CAD build for the part. Positions are in the model's coordinates, mm. Face numbers are marked on the shaded views. A direction names the side the tool comes from. Give positions to 0.01 mm unless a question says otherwise; leave off trailing zeros. Order: outer loops, then holes, each group sorted by start corner. A loop starts at its lowest first (then second) coordinate and runs counter-clockwise, first axis right, second up.
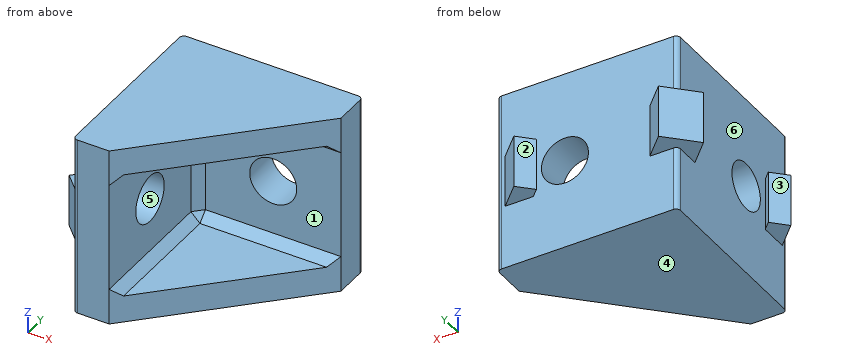
```python
from build123d import *

# Parameters (mm, degrees)
EXTRUDE_1_DEPTH     = 10
EXTRUDE_2_DEPTH     = 3
SKETCH_3_R          = 2.6
CUT_EXTRUDE_1_DEPTH = 25.738633754
SKETCH_4_R          = 2.6
CUT_EXTRUDE_2_DEPTH = 25.738633754
EXTRUDE_START       = -10
EXTRUDE_3_DEPTH     = 2.9
FILLET_1_R          = 0.5
CHAMFER_1_SIZE      = 1


with BuildPart() as part:
    # Эскиз1 → Бобышка-Вытянуть1 (new, symmetric)
    with BuildSketch(Plane.XY):
        Polygon((0, 0), (0, -16), (-4, -16), (-4, 4), (16, 4), (16, 0), align=None)
    extrude(amount=EXTRUDE_1_DEPTH, both=True)

    # Эскиз2 → Бобышка-Вытянуть2 (add)
    with BuildSketch(Plane.XY.offset(10)):
        Polygon((0, -16), (0, 0), (16, 0), align=None)
    extrude_2 = extrude(amount=-EXTRUDE_2_DEPTH)

    # Зеркальное отражение1: Бобышка-Вытянуть2 across plane
    add(extrude_2.mirror(Plane.XY))

    # Эскиз3 → Вырез-Вытянуть1 (cut, through all)
    with BuildSketch(Plane(origin=(0, 0, 0), x_dir=(0, 0, -1), z_dir=(1, 0, 0))):
        with Locations((0, -8.5)):
            Circle(SKETCH_3_R)
        with Locations((20, -8.5)):
            Circle(SKETCH_3_R)
        with Locations((20, 11.5)):
            Circle(SKETCH_3_R)
        with Locations((0, 11.5)):
            Circle(SKETCH_3_R)
    extrude(amount=-CUT_EXTRUDE_1_DEPTH, mode=Mode.SUBTRACT)

    # Эскиз4 → Вырез-Вытянуть2 (cut, through all)
    with BuildSketch(Plane.XZ):
        with Locations((8.5, 0)):
            Circle(SKETCH_4_R)
        with Locations((-11.5, 0)):
            Circle(SKETCH_4_R)
        with Locations((-11.5, 20)):
            Circle(SKETCH_4_R)
        with Locations((8.5, 20)):
            Circle(SKETCH_4_R)
    extrude(amount=-CUT_EXTRUDE_2_DEPTH, mode=Mode.SUBTRACT)

    # Эскиз5 → Бобышка-Вытянуть3 (add, symmetric)
    with BuildSketch(Plane.XY.offset(10).offset(EXTRUDE_START)):
        Polygon((-0.888730163, 4), (-3.292893219, 6.404163056), (-6.404163056, 3.292893219), (-4, 0.888730163), (-4, 4), align=None)
        Polygon((16, 3.111269837), (12.707106781, 6.404163056), (11.151471863, 4.848528137), (16, 0), align=None)
        Polygon((-4.848528137, -11.151471863), (0, -16), (-3.111269837, -16), (-6.404163056, -12.707106781), align=None)
    extrude(amount=EXTRUDE_3_DEPTH, both=True)

    # Скругление1
    fillet_1_edges = [part.edges().sort_by_distance(p)[0] for p in [
        (-4, -16, 0),
        (-4, 4, 6.45),
        (16, 4, 0),
        (-4, 4, -6.45),
    ]]
    fillet(fillet_1_edges, radius=FILLET_1_R)

    # Фаска1
    chamfer_1_edges = [part.edges().sort_by_distance(p)[0] for p in [
        (0, 0, 0),
        (0, -8, 7),
        (8, 0, 7),
        (8, 0, -7),
        (0, -8, -7),
    ]]
    chamfer(chamfer_1_edges, length=CHAMFER_1_SIZE)


solid = part.part
```
Item 1: Tool access for the marked faces 1, 2 and 3: list every direction of +Z, -Z, +X, -X, +Y, -Y with a clear straight run to the whole face (end or side of a thin tool).
Item 2: Slice it at B-B (z = 1). Give the cut face in (x, y).
Item 3: Drop flat-ended pins along their axis: pin 1 Ø4 at (x, z) = (6, -8) entering from +Y; pin 2 Ø0.7 at (x, y) = (13, 5.5) entering from -Z; pin 3 Ø8 at (y, z) = (-6, 6) entering from +X. Give the stop position or say it passes through.
Item 4: Two-plate mould, pull along Z, no slides. Class the marked faces 4, 5 and 6: released by +Z, released by -Z, zero draft, split by the parting line, or undercut.
Item 5: Wall check: L1, parallel to Y at x = -0.85, z = 0; L2, parallel to Z at x = 8.5, y = 2.75; L3, parallel to Z at x = 10.75, y = -3.75. Give the ranges that are in metal, low to high.
Item 6: Slice it at A-A (x = 8.5). Give the cut face in (y, z), and give its area (3 significant figures).
Item 7: Slice it at D-D (y = -4). Give the cut face in (x, z), and give its area (3 significant figures).
Item 8: Slice it at C-C (y = -8.5). Give the cut face in (x, z), and give its area (3 significant figures).
A:
1. face 1: +X, -Y
1. face 2: +Z, -Z, +Y
1. face 3: +Z, -Z, -X
2. outline: (-6.4, -12.71) - (-4, -15.11) - (-4, -15.5) arc R0.5 ccw to (-3.5, -16) - (0, -16) - (0, -10.9) - (-4, -10.9) - (-4, -12) - (-4.85, -11.15) - close; (-6.4, 3.29) - (-4, 0.89) - (-4, -6.1) - (0, -6.1) - (0, -1) - (1, 0) - (6.1, 0) - (6.1, 4) - (-0.89, 4) - (-3.29, 6.4) - close; (10.9, 0) - (16, 0) - (16, 3.5) arc R0.5 ccw to (15.5, 4) - (15.11, 4) - (12.71, 6.4) - (11.15, 4.85) - (12, 4) - (10.9, 4) - close
3. pin 1: stops at y = 4
3. pin 2: stops at z = -2.9
3. pin 3: stops at x = 13.87
4. face 4: released by -Z
4. face 5: undercut
4. face 6: zero draft
5. L1: y = -16 to -11.1, -5.9 to 4
5. L2: z = -10 to -2.6, 2.6 to 10
5. L3: z = -10 to -7, 7 to 10
6. outline: (-7.5, -10) - (4, -10) - (4, -2.6) - (0, -2.6) - (0, -6) - (-1, -7) - (-7.5, -7) - close; (-7.5, 7) - (-1, 7) - (0, 6) - (0, 2.6) - (4, 2.6) - (4, 10) - (-7.5, 10) - close
6. area: 105 mm2
7. outline: (-4, -10) - (12, -10) - (12, -7) - (1, -7) - (0, -6) - (0, 6) - (1, 7) - (12, 7) - (12, 10) - (-4, 10) - close
7. area: 153 mm2
8. outline: (-4, -10) - (7.5, -10) - (7.5, -7) - (1, -7) - (0, -6) - (0, -2.6) - (-4, -2.6) - close; (-4, 2.6) - (0, 2.6) - (0, 6) - (1, 7) - (7.5, 7) - (7.5, 10) - (-4, 10) - close
8. area: 105 mm2
